Read the model definition and answer for the solid it produces. Units are mm, in the model's axes. A direction names the side the tool comes from. Give positions to 0.01 mm unless a question says otherwise; leave off trailing zeros. Order: outer loops, then holes, each group sorted by start corner. A loop starts at its lowest first (then second) coordinate and runs counter-clockwise, first axis right, second up. Notation, with made-up numbers: (26.5, -8) - (76.5, -8) arc R19 cw to (76.5, 21) - close; hole circle Ø2 at (1, 60.5). An arc over 180 degrees is marked (long way). One line per item, written item: value. Start each with the question number.
```python
from build123d import *

# Parameters (mm, degrees)
BOSS_EXTRU_1_DEPTH      = 160
ESQUISSE2_W             = 18
ESQUISSE2_H             = 18
ENL_V_MAT_EXTRU_1_DEPTH = 3
ESQUISSE6_R             = 1.4
ENL_V_MAT_EXTRU_5_DEPTH = 3


with BuildPart() as part:
    # Esquisse1 → Boss.-Extru.1 (new body)
    with BuildSketch(Plane.XY):
        Polygon((0, 0), (20, 0), (20, 2), (2, 2), (2, 20), (0, 20), align=None)
    extrude(amount=BOSS_EXTRU_1_DEPTH)

    # Esquisse2 → Enlèv. mat.-Extru.1 (cut, through all)
    with BuildSketch(Plane(origin=(2, 0, 0), x_dir=(0, 0, -1), z_dir=(1, 0, 0))):
        with Locations((-151, 11)):
            Rectangle(ESQUISSE2_W, ESQUISSE2_H)
        with Locations((-9, 11)):
            Rectangle(ESQUISSE2_W, ESQUISSE2_H)
    extrude(amount=-ENL_V_MAT_EXTRU_1_DEPTH, mode=Mode.SUBTRACT)

    # Esquisse6 → Enlèv. mat.-Extru.5 (cut, through all)
    with BuildSketch(Plane(origin=(0, 2, 0), x_dir=(1, 0, 0), z_dir=(0, 1, 0))):
        with Locations((6.48, -145.52)):
            Circle(ESQUISSE6_R)
        with Locations((6.48, -14.48)):
            Circle(ESQUISSE6_R)
        with Locations((16.48, -155.52)):
            Circle(ESQUISSE6_R)
        with Locations((16.48, -4.48)):
            Circle(ESQUISSE6_R)
    extrude(amount=-ENL_V_MAT_EXTRU_5_DEPTH, mode=Mode.SUBTRACT)


solid = part.part
```
1) The mould has two halves that part along X. Classify faces 3 (the flat face through (10, 2, 81)), 4 (the cylindrical face through (6.3, 1.01, 144.13)), 5 (the flat face through (0, 10, 79)): +X half, -X half, draft (parallel to the pull), parting line (faces both ways), or undercut.
2) Section D-D on y = 16.25 is taken. Write down the section's boundary in (x, z), plus the area to 3 significant figures.
3) Each of these flat-tipped pins is pushed along its axis until it touches: pin 1 (4.5 mm diameter, centred on x = 6.48, z = 145.52, fed in from +Y); pin 2 (12 mm diameter, centred on y = 10, z = 132, fed in from +X); pin 3 (6 mm diameter, centred on x = 8, y = 6.5, fed in from -Z); pin 4 (0.6 mm diameter, centred on x = 0.5, y = 8, fed in from -Z). Where does it stop, or does it pass through?
4) Section A-A on z = 14.48 is taken. Write down the section's boundary in (x, y), plus the area to 3 significant figures.
5) For faces 1 (the flat face through (2, 11, 79)), 2 (the cylindrical face through (6.177, 1.014, 15.847)), determine the directions among +Z, -Z, +X, -X, +Y, -Y from which every point of the face is accessible in a straight line to the end or side of a thin tool.
6) Section B-B on x = 16.48 is taken. Write down the section's boundary in (y, z), plus the area to 3 significant figures.
7) Section C-C on z = 47.5 is taken. Write down the section's boundary in (x, y).
8) Find the intervals of material crossed by probe 1 along Z at (x, y) = (6.48, 0.55); probe 2 along Z at (x, y) = (16.48, 1); probe 3 along X at (y, z) = (0.85, 14.48), in increasing order. Write a range as from..to.
Solved:
1. face 3: draft
1. face 4: undercut
1. face 5: -X half
2. outline: (0, 18) - (2, 18) - (2, 142) - (0, 142) - close
2. area: 248 mm2
3. pin 1: stops at y = 2
3. pin 2: stops at x = 2
3. pin 3: passes through
3. pin 4: stops at z = 18
4. outline: (0, 0) - (5.08, 0) - (5.08, 2) - (0, 2) - close; (7.88, 0) - (20, 0) - (20, 2) - (7.88, 2) - close
4. area: 34.4 mm2
5. face 1: +Z, -Z, +X, +Y
5. face 2: +Y, -Y
6. outline: (0, 0) - (2, 0) - (2, 3.08) - (0, 3.08) - close; (0, 5.88) - (2, 5.88) - (2, 154.12) - (0, 154.12) - close; (0, 156.92) - (2, 156.92) - (2, 160) - (0, 160) - close
6. area: 309 mm2
7. outline: (0, 0) - (20, 0) - (20, 2) - (2, 2) - (2, 20) - (0, 20) - close
8. probe 1: z = 0..13.08, 15.88..144.12, 146.92..160
8. probe 2: z = 0..3.08, 5.88..154.12, 156.92..160
8. probe 3: x = 0..5.08, 7.88..20
